Input: part model. Units: mm. Frame: model coordinates. Face numbers are marked on the shaded views. A direction names the side the tool comes from. Give positions to 0.01 mm unless a question says otherwise; leave off trailing zeros. Write each loop counter-clockwise with the first axis right and the second up, starting at its lowest first coordinate (ties: lowest second). Pieces come first, ordered by that corner, then holes. Notation, with made-up numbers: (32.5, 2) -> (41.5, 2) arc R3 ccw to (41.5, 7) -> close; hole circle Ø2 at (-17, -9). An arc over 180 degrees is marked (long way). Return JSON: item names as keys, results as strings. Group by question number.
Item 1: Section D-D, the plane x = 8. Return loops of the section in (y, z).
Item 2: Section A-A, the plane z = 12.5. Return loops of the section in (x, y).
Item 3: Section B-B, the plane x = -7.5. Return loops of the section in (y, z), then the cut area to 3 significant figures.
Item 4: Set-up query: the marked faces 1, 2 and 3. Return all of +Z, -Z, +X, -X, +Y, -Y with unobstructed straight access to the full face (end or side cutting, diameter ignored); none if empty.
Item 5: Section C-C, the plane y = 8. Return loops of the section in (x, z), then the cut area to 3 significant figures.
Item 6: Pin query (flat end, axial travel): P1, Ø5, axis at x = -12.5, y = 6, coming from the -Z side; P2, Ø1.5, axis at y = 1.5, z = -5, coming from the +X side; P3, Ø5, axis at x = -14, y = 6, coming from the +Z side. Return the tip coordinate at first contact, or that it passes through.
Item 7: Line query: line 1 (Z direction, x = 3.75, y = 5); line 2 (Z direction, x = 6.25, y = 7.25); line 3 (X direction, y = 9.25, z = -8.5). Output: solid intervals per line, ascending. Write a range as [from, to].
Item 8: Mould query, pull axis Z, two halves, no side actions, for the marked faces 4, 5 and 6. Classes: released by +Z, released by -Z, zero draft, split by the parting line, or undercut.
from build123d import *

# Parameters (mm, degrees)
SKETCH_1_R      = 1.25
EXTRUDE_1_DEPTH = 10


with BuildPart() as part:
    # 草圖1 → 填料-伸長1 (new body)
    with BuildSketch(Plane(origin=(0, 0, 0), x_dir=(1, 0, 0), z_dir=(0, 1, 0))):
        with BuildLine():
            Line((0.155444566, 5.269237886), (6.404504741, 16.092927609))
            ThreePointArc((6.404504741, 16.092927609), (5.191725275, 16.524103264), (3.950274568, 16.864024752))
            ThreePointArc((3.950274568, 16.864024752), (-4.820507676, 8.349364213), (-16.579811129, 5.010974248))
            ThreePointArc((-16.579811129, 5.010974248), (-16.906155839, 3.765885654), (-17.139136501, 2.5))
            Line((-17.139136501, 2.5), (-4.641016151, 2.5))
            ThreePointArc((-4.641016151, 2.5), (-2.141016151, 0), (-4.641016151, -2.5))
            Line((-4.641016151, -2.5), (-17.139136501, -2.5))
            ThreePointArc((-17.139136501, -2.5), (-16.906155839, -3.765885654), (-16.579811129, -5.010974248))
            ThreePointArc((-16.579811129, -5.010974248), (-4.820507676, -8.349364213), (3.950274568, -16.864024752))
            ThreePointArc((3.950274568, -16.864024752), (5.191725275, -16.524103264), (6.404504741, -16.092927609))
            Line((6.404504741, -16.092927609), (0.155444566, -5.269237886))
            ThreePointArc((0.155444566, -5.269237886), (1.070508076, -1.854174377), (4.485571585, -2.769237886))
            Line((4.485571585, -2.769237886), (10.73463176, -13.592927609))
            ThreePointArc((10.73463176, -13.592927609), (11.714430563, -12.75821761), (12.629536561, -11.853050504))
            ThreePointArc((12.629536561, -11.853050504), (9.641015352, 0), (12.629536561, 11.853050504))
            ThreePointArc((12.629536561, 11.853050504), (11.714430563, 12.75821761), (10.73463176, 13.592927609))
            Line((10.73463176, 13.592927609), (4.485571585, 2.769237886))
            ThreePointArc((4.485571585, 2.769237886), (1.070508076, 1.854174377), (0.155444566, 5.269237886))
        make_face()
        with Locations(Location((0.048558271, 0.050271222, 0), (0, 0, 270))):
            Circle(SKETCH_1_R, mode=Mode.SUBTRACT)
    extrude(amount=EXTRUDE_1_DEPTH)


solid = part.part
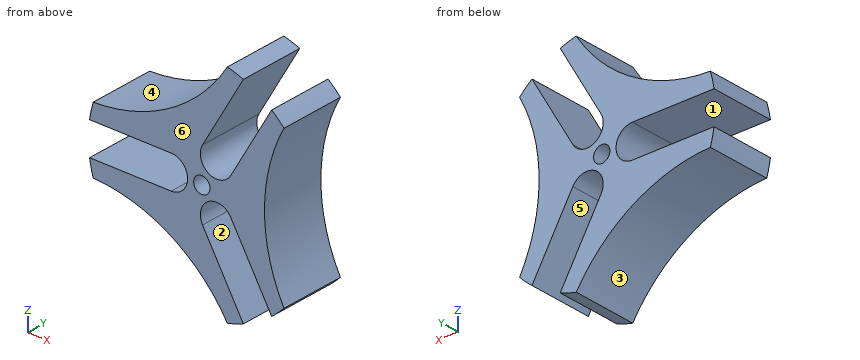
Answer below:
{
 "1": {"outline": "(0, -8.86) -> (10, -8.86) -> (10, 8.86) -> (0, 8.86) -> close"},
 "2": {"outline": "(0.53, 0) -> (4.33, 0) -> (4.33, 10) -> (0.53, 10) -> close; (10.1, 0) -> (11.99, 0) -> (11.99, 10) -> (10.1, 10) -> close"},
 "3": {"outline": "(0, -7.01) -> (10, -7.01) -> (10, -2.5) -> (0, -2.5) -> close; (0, 2.5) -> (10, 2.5) -> (10, 7.01) -> (0, 7.01) -> close", "area": "90.2 mm2"},
 "4": {"face 1": "-X, +Y, -Y", "face 2": "+Y, -Y", "face 3": "-Z, -X, +Y, -Y"},
 "5": {"outline": "(-17.14, -2.5) arc R17.32 ccw to (-16.58, -5.01) arc R25 cw to (3.95, -16.86) arc R17.32 ccw to (6.4, -16.09) -> (0.16, -5.27) arc R2.5 cw to (4.49, -2.77) -> (10.73, -13.59) arc R17.32 ccw to (12.63, -11.85) arc R25 cw to (12.63, 11.85) arc R17.32 ccw to (10.73, 13.59) -> (4.49, 2.77) arc R2.5 cw to (0.16, 5.27) -> (6.4, 16.09) arc R17.32 ccw to (3.95, 16.86) arc R25 cw to (-16.58, 5.01) arc R17.32 ccw to (-17.14, 2.5) -> (-4.64, 2.5) arc R2.5 cw to (-4.64, -2.5) -> close; hole circle Ø2.5 at (0.05, -0.05)", "area": "346 mm2"},
 "6": {"P1": "stops at z = -6.1", "P2": "stops at x = 10.31", "P3": "stops at z = 5.69"},
 "7": {"line 1": "z = [-16.55, -11.5], [-1.97, 1.97], [11.5, 16.55]", "line 2": "z = [-16.15, -15.83], [-5.83, 5.83], [15.83, 16.15]", "line 3": "x = [-4.56, 2.02], [7.79, 11.13]"},
 "8": {"face 4": "released by +Z", "face 5": "undercut", "face 6": "zero draft"}
}
